Autodesk Inventor part; units mm, degrees
ref_plane "YZ Plane" through (0, 0, 0) normal (1, 0, 0) x (0, 1, 0)
ref_plane "XZ Plane" through (0, 0, 0) normal (0, 1, 0) x (-1, 0, 0)
ref_plane "XY Plane" through (0, 0, 0) normal (0, 0, 1) x (1, 0, 0)
sketch "Sketch1" plane through (0, 0, 0) normal (0, 1, 0) x (-1, 0, 0)
  line L0 (0.7432, 9.5847) -> (-0.7568, 9.5847)
  line L1 (-0.7568, 9.5847) -> (-0.7568, -10.4153)
  line L2 (-0.7568, -10.4153) -> (0.7432, -10.4153)
  line L3 (0.7432, -10.4153) -> (0.7432, 9.5847)
  point P0 (0, 0)
  dimension "d0" = 20
  dimension "d1" = 1.5
extrude "Extrusion1" add sketch "Sketch1" along normal blind 50
sketch "Sketch2" plane through (0, 0, 0) normal (0, -1, 0) x (1, 0, 0)
  point P0 (0, 0)
sketch "Sketch3" plane through (0, 0, 0) normal (0, -1, 0) x (1, 0, 0)
  line L0 (-0.7432, -10.4153) -> (-0.7432, 9.5847)
  line L1 (0.7568, 9.5847) -> (0.7568, -10.4153)
  line L2 (-0.7432, 6.59) -> (0.7568, 6.59)
  line L3 (0.7568, 6.59) -> (0.7568, 1.59)
  line L4 (0.7568, 1.59) -> (-0.7432, 1.59)
  line L5 (-0.7432, 1.59) -> (-0.7432, 6.59)
  line L6 (-0.7432, -2.11) -> (0.7568, -2.11)
  line L7 (0.7568, -2.11) -> (0.7568, -7.11)
  line L8 (0.7568, -7.11) -> (-0.7432, -7.11)
  line L9 (-0.7432, -7.11) -> (-0.7432, -2.11)
  point P0 (0, 0)
  point P1 (-0.7432, -7.11)
  point P2 (0.7568, -2.11)
  dimension "d4" = 5
  dimension "d5" = 5
extrude "Extrusion2" add sketch "Sketch3" along normal blind 5 contours L0 L6 L1 L8
properties part number "Arcylic_Panel_Base_20mm_P2"
Geometry: final body of the model. Coordinates: model frame, mm. A direction names the side the tool comes from. Coordinates: 2 decimals unless noted, no trailing zeros. Order: outer loops, then holes, each group sorted by start corner. A loop starts at its lowest first (then second) coordinate and runs counter-clockwise, first axis right, second up. Notation, with made-up numbers: M -13,6.5 L 23,6.5 A17 cw 23,34.5 Z; hole C 88,-37 d11. An arc over 180 degrees is marked long. Answer in a Markdown table with one row per item. Add a question column.
Q1. Section query B-B on z = -1.5. Return the cut outline in (x, y).
Q2. Line query: L1, parallel to Y at x = -0.4, z = 6.75. Output: solid intervals per line, ascending.
Q3. Section query A-A on x = -0.4. Return the cut outline in (y, z).
Q4. Reachability of faces 1 (the flat face through (0, -2, -2.11)), 2 (the flat face through (0, 50, 0)), 3 (the flat face through (0, 0, -9)) from +Z, -Z, +X, -X, +Y, -Y: full face, straight path, thin tool, end or side. Return the list, or none.
Completed:
| question | item | result |
|---|---|---|
| 1 | outline | M -0.74,0 L 0.76,0 L 0.76,50 L -0.74,50 Z |
| 2 | L1 | y = 0 to 50 |
| 3 | outline | M -5,-7.11 L 0,-7.11 L 0,-10.42 L 50,-10.42 L 50,9.58 L 0,9.58 L 0,-2.11 L -5,-2.11 Z |
| 4 | face 1 | +Z, +X, -X, -Y |
| 4 | face 2 | +Z, -Z, +X, -X, +Y |
| 4 | face 3 | -Z, +X, -X, -Y |
